Design review of the part built by this model. Coordinates are the model's own, in mm. A direction names the side the tool comes from. Give positions to 0.01 mm unless a question says otherwise; leave off trailing zeros. Write each loop counter-clockwise with the first axis right and the second up, starting at its lowest first coordinate (ties: lowest second). Pieces come first, ordered by that corner, then holes. Notation, with made-up numbers: M 14,-39.75 L 18,-39.75 A35 ccw 18,-6.75 Z; hole C 69,-39 d6. An arc over 180 degrees is marked long. Answer in a Markdown table with one row per item.
```python
from build123d import *

# Parameters (mm, degrees)
SKETCH1_R           = 4.5
BOSS_EXTRUDE1_DEPTH = 1.1


with BuildPart() as part:
    # Sketch1 → Boss-Extrude1 (new body)
    with BuildSketch(Plane.XY):
        with BuildLine():
            Line((-9.5, -60), (-9.5, 0))
            ThreePointArc((-9.5, 0), (-6.717514421, 6.717514421), (0, 9.5))
            Line((0, 9.5), (60, 9.5))
            ThreePointArc((60, 9.5), (69.272242002, 2.067735054), (64.036324171, -8.599888789))
            ThreePointArc((64.036324171, -8.599888789), (31.466251763, -31.466251763), (8.599888789, -64.036324171))
            ThreePointArc((8.599888789, -64.036324171), (-2.067735054, -69.272242002), (-9.5, -60))
        make_face()
        Circle(SKETCH1_R, mode=Mode.SUBTRACT)
        with BuildLine():
            Line((-4.5, -60), (-4.5, -54))
            ThreePointArc((-4.5, -54), (0, -49.5), (4.5, -54))
            Line((4.5, -54), (4.5, -60))
            ThreePointArc((4.5, -60), (0, -64.5), (-4.5, -60))
        make_face(mode=Mode.SUBTRACT)
        with BuildLine():
            Line((60, -4.5), (54, -4.5))
            ThreePointArc((54, -4.5), (49.5, 0), (54, 4.5))
            Line((54, 4.5), (60, 4.5))
            ThreePointArc((60, 4.5), (64.5, 0), (60, -4.5))
        make_face(mode=Mode.SUBTRACT)
    extrude(amount=-BOSS_EXTRUDE1_DEPTH)


solid = part.part
```
1) The part is to be moulded in two halves that separate along Y. For faces 1 (the face through (22, -21, 0)), 2 (the face through (-0.59, 4.46, -0.54)), 3 (the face through (64.5, 0.1, -0.5)), 4 (the face through (-1.89, -69.31, -0.54)), say which applies: released by +Y, released by -Y, zero draft, split by the parting line, or undercut.
Geometry says:
| item | result |
|---|---|
| face 1 | zero draft |
| face 2 | undercut |
| face 3 | undercut |
| face 4 | released by -Y |
2) Add section A-A (z = -0.7). Write out the cut boundary in (x, y).
Geometry says:
| item | result |
|---|---|
| outline | M -9.5,-60 A9.5 ccw 8.6,-64.04 A115.4 cw 64.04,-8.6 A9.5 ccw 60,9.5 L 0,9.5 A9.5 ccw -9.5,0 Z; hole M -4.5,-60 A4.5 ccw 4.5,-60 L 4.5,-54 A4.5 ccw -4.5,-54 Z; hole C 0,0 d9; hole M 54,-4.5 L 60,-4.5 A4.5 ccw 60,4.5 L 54,4.5 A4.5 ccw Z |
3) Insertion check: P1, Ø10.5, axis at x = 0, y = 0, coming from the +Z side. The pin has a flat end and moves straight along its axis. Give the tip position at first contact, or say it passes through.
Geometry says:
| item | result |
|---|---|
| P1 | z = 0 |
4) Add section D-D (y = -20). Write out the cut boundary in (x, z).
Geometry says:
| item | result |
|---|---|
| outline | M -9.5,-1.1 L 44.83,-1.1 L 44.83,0 L -9.5,0 Z |
5) To check wall thickness, follow probe 1 along Y at (x, z) = (0, -0.55); probe 2 along Y at (x, z) = (4, -0.9); probe 3 along X at (y, z) = (4, -0.15). State the ranges of each line that lie inside material, in increasing order. Write a range as [from, to].
Geometry says:
| item | result |
|---|---|
| probe 1 | [-69.5, -64.5], [-49.5, -4.5], [4.5, 9.5] |
| probe 2 | [-68.62, -62.06], [-51.94, -2.06], [2.06, 9.5] |
| probe 3 | [-8.62, -2.06], [2.06, 51.94], [62.06, 68.62] |
6) Add section B-B (y = -50.5). Write out the cut boundary in (x, z), and give its area (3 significant figures).
Geometry says:
| item | result |
|---|---|
| outline | M -9.5,-1.1 L -2.83,-1.1 L -2.83,0 L -9.5,0 Z; M 2.83,-1.1 L 16.1,-1.1 L 16.1,0 L 2.83,0 Z |
| area | 21.9 mm^2 |
7) Add section C-C (x = 1). Write out the cut boundary in (y, z), and give its area (3 significant figures).
Geometry says:
| item | result |
|---|---|
| outline | M -69.45,-1.1 L -64.39,-1.1 L -64.39,0 L -69.45,0 Z; M -49.61,-1.1 L -4.39,-1.1 L -4.39,0 L -49.61,0 Z; M 4.39,-1.1 L 9.5,-1.1 L 9.5,0 L 4.39,0 Z |
| area | 60.9 mm^2 |
8) For faces 5 (the face through (69.231, 2.243, -0.542)), 6 (the face through (0.1, -64.5, -0.5)), list the 3-axis set-ups (+Z, -Z, +X, -X, +Y, -Y) from which the entire face can be reached by the end or side of a thin tool; tool diameter is ignored.
Geometry says:
| item | result |
|---|---|
| face 5 | +Z, -Z, +X |
| face 6 | +Z, -Z |
